Verification items for this drawing (mm, ordinates from the low corner). A direction names the side the tool comes from. Round coordinates to 2 decimals unless told otherwise and drop trailing zeros. Order: outer loops, then holes, each group sorted by start corner. A loop starts at its lowest first (then second) coordinate and runs counter-clockwise, first axis right, second up. Notation, with made-up numbers: (9, 83) -> (31, 83) arc R30 ccw to (31, 116) -> close; hole circle Ø2 at (17.25, -10.5). An arc over 180 degrees is marked (long way). Answer in a Markdown table with one row per item. Add a question column.
1. Sectioned sample at A-A, the plane y = 14. Record the boundary of the cut face in (x, z), then the cut area to 3 significant figures.
2. Sectioned sample at B-B, the plane z = 6.75. Record the boundary of the cut face in (x, y), then the cut area to 3 significant figures.
3. Sectioned sample at D-D, the plane x = 27.5. Record the boundary of the cut face in (y, z), then the cut area to 3 significant figures.
4. Material ranges on L1, parallel to Y at x = 27.5, z = 17.25; L2, parallel to X at y = 8, z = 17.5; L3, parallel to Y at x = 37, z = 16.55, recorded low to high. Write a range as from..to.
5. Sectioned sample at C-C, the plane x = 37. Record the boundary of the cut face in (y, z), then the cut area to 3 significant figures.
6. Draft check along Y on the marked faces 1, 2 and 3. Enter one of: +Y half, -Y half, draft (parallel to the pull), parting line (faces both ways), or undercut.
7. Access from +Z, -Z, +X, -X, +Y, -Y to the whole of each face (thin tool, end or side, straight path). Record for the marked faces 4, 5 and 6.
8. Depth check by flat-ended pin: P1, Ø4, axis at y = 18.5, z = 11, coming from the +X side; P2, Ø1.5, axis at y = 32.5, z = 14, coming from the -X side; P3, Ø6, axis at x = 34, y = 19.5, coming from the -Z side. Enter the tip coordinate at first touch or a pass-through.
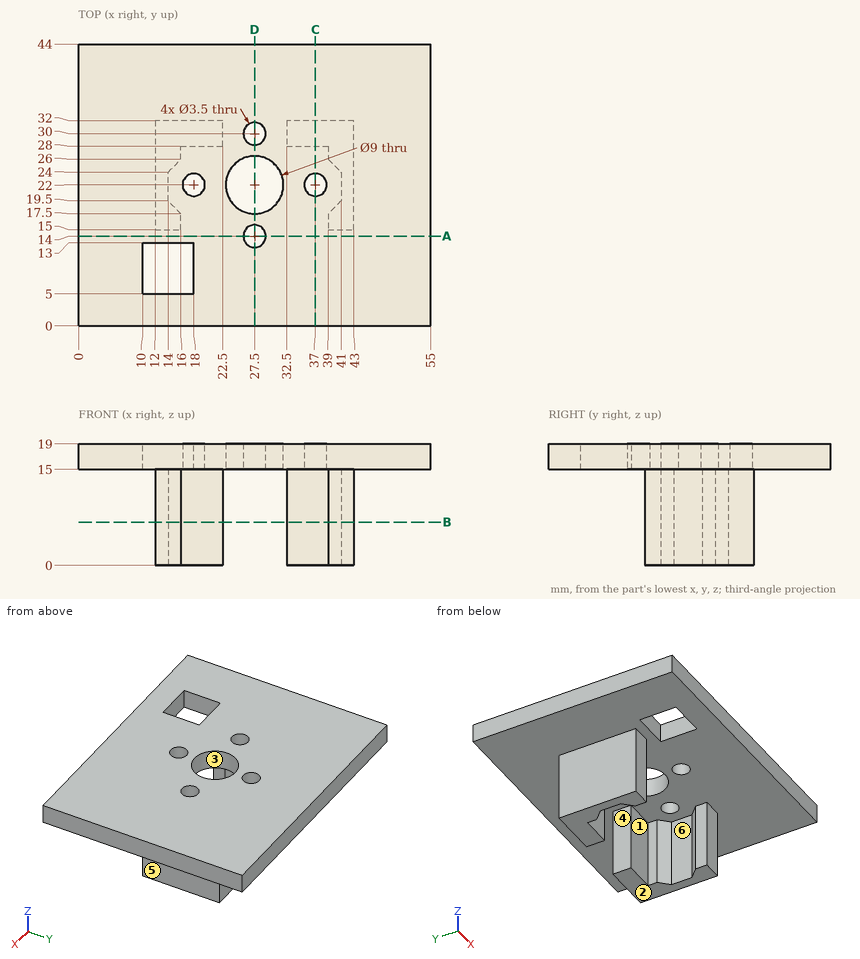
Answer key:
| question | item | result |
|---|---|---|
| 1 | outline | (0, 15) -> (25.75, 15) -> (25.75, 19) -> (0, 19) -> close; (29.25, 15) -> (55, 15) -> (55, 19) -> (29.25, 19) -> close |
| 1 | area | 206 mm² |
| 2 | outline | (12, 15) -> (16, 15) -> (16, 17.5) -> (14, 19.5) -> (14, 24) -> (16, 26) -> (16, 28) -> (22.5, 28) -> (22.5, 32) -> (12, 32) -> close; (32.5, 28) -> (39, 28) -> (39, 26) -> (41, 24) -> (41, 19.5) -> (39, 17.5) -> (39, 15) -> (43, 15) -> (43, 32) -> (32.5, 32) -> close |
| 2 | area | 162 mm² |
| 3 | outline | (0, 15) -> (12.25, 15) -> (12.25, 19) -> (0, 19) -> close; (15.75, 15) -> (17.5, 15) -> (17.5, 19) -> (15.75, 19) -> close; (26.5, 15) -> (28.25, 15) -> (28.25, 19) -> (26.5, 19) -> close; (31.75, 15) -> (44, 15) -> (44, 19) -> (31.75, 19) -> close |
| 3 | area | 112 mm² |
| 4 | L1 | y = 0..12.25, 15.75..17.5, 26.5..28.25, 31.75..44 |
| 4 | L2 | x = 0..10, 18..55 |
| 4 | L3 | y = 0..20.25, 23.75..44 |
| 5 | outline | (0, 15) -> (20.25, 15) -> (20.25, 19) -> (0, 19) -> close; (23.75, 15) -> (28, 15) -> (28, 0) -> (32, 0) -> (32, 15) -> (44, 15) -> (44, 19) -> (23.75, 19) -> close |
| 5 | area | 222 mm² |
| 6 | face 1 | -Y half |
| 6 | face 2 | draft |
| 6 | face 3 | undercut |
| 7 | face 4 | -Z, +Y, -Y |
| 7 | face 5 | -Z, +X, +Y, -Y |
| 7 | face 6 | -Z |
| 8 | P1 | stops at x = 43 |
| 8 | P2 | stops at x = 12 |
| 8 | P3 | stops at z = 15 |
